Autodesk Inventor part; units mm, degrees
ref_plane "YZ Plane" through (0, 0, 0) normal (1, 0, 0) x (0, 1, 0)
ref_plane "XZ Plane" through (0, 0, 0) normal (0, 1, 0) x (-1, 0, 0)
ref_plane "XY Plane" through (0, 0, 0) normal (0, 0, 1) x (1, 0, 0)
sketch "Эскиз1" plane through (0, 0, 0) normal (0, 0, 1) x (1, 0, 0)
  line L0 (0, 0) -> (10, 0)
  line L1 (10, 0) -> (10, 30)
  line L2 (10, 30) -> (0, 30)
  line L3 (0, 30) -> (0, 0)
  dimension "d0" = 10
  dimension "d1" = 30
revolve "Вращение1" add sketch "Эскиз1" angle 360 about axis through (0, 0, 0) along (1, 0, 0)
sketch "Эскиз2" plane through (0, 0, 0) normal (0, 0, 1) x (1, 0, 0)
  line L0 (0, 0) -> (10, 0)
  line L1 (10, -30) -> (10, 30)
  arc A0 (3, 20) -> (0, 23) centre (0, 20) ccw
  line L2 (3, 20) -> (0, 20) construction
  line L3 (0, 23) -> (0, 20) construction
  line L4 (7, 20) -> (7, 10)
  arc A1 (7, 6) -> (10, 3) centre (10, 6) ccw
  line L5 (7, 6) -> (10, 6) construction
  line L6 (10, 3) -> (10, 6) construction
  arc A2 (10, 23) -> (7, 20) centre (10, 20) ccw
  line L7 (7, 20) -> (10, 20) construction
  line L8 (10, 23) -> (10, 20) construction
  line L9 (7, 10) -> (7, 6)
  line L10 (0, -30) -> (0, 30)
  line L11 (0, 0) -> (0, 23)
  line L12 (10, 3) -> (10, 23)
  line L13 (3, 20) -> (3, 0)
  point P0 (10, 3)
  point P1 (10, 23)
  dimension "d4" = 3
  dimension "d5" = 90
  dimension "d6" = 3
  dimension "d7" = 90
  dimension "d8" = 3
  dimension "d9" = 90
  dimension "d10" = 3
  dimension "d12" = 20
  dimension "d14" = 20
revolve "Вращение2" cut sketch "Эскиз2" angle 360 about axis through (0, 0, 0) along (-1, 0, 0) contours A1 L9 L4 A2 L1
sketch "Эскиз3" plane through (10, 0, 0) normal (1, 0, 0) x (0, 0, -1)
  point P0 (0, 0)
  point P1 (26.5, 0)
  point P2 (13.25, 22.9497)
  point P3 (-13.25, 22.9497)
  point P4 (-26.5, 0)
  point P5 (-13.25, -22.9497)
  point P6 (13.25, -22.9497)
  dimension "d15" = 26.5
  dimension "d18" = 360
hole "Отверстие1" at (10, 0, -26.5) at (10, 22.9497, -13.25) at (10, 22.9497, 13.25) at (10, 0, 26.5) at (10, -22.9497, 13.25) at (10, -22.9497, -13.25) direction (-1, 0, 0) diameter 4 end through all
sketch "Эскиз4" plane through (0, 0, 0) normal (0, 0, 1) x (1, 0, 0)
  line L0 (0, 0) -> (10, 0)
  line L1 (10, 2) -> (10, -2)
  line L2 (0, 0) -> (3, 0)
  line L3 (3, 0) -> (3, 20)
  line L4 (0, 23) -> (0, 23)
  line L5 (0, 23) -> (0, 0)
  arc A0 (10, 23) -> (7, 20) centre (10, 20) ccw construction
  arc A1 (3, 20) -> (0, 23) centre (0, 20) ccw
  dimension "d29" = 3
revolve "Вращение3" cut sketch "Эскиз4" angle 360 about axis through (0, 0, 0) along (1, 0, 0)
equation "\"d25\" = d15"
properties part number "711126 (Доделать)"
Design review of the part built by this model. Coordinates are the model's own, in mm. A direction names the side the tool comes from. Round coordinates to 2 decimals unless told otherwise and drop trailing zeros. Write each loop counter-clockwise with the first axis right and the second up, starting at its lowest first coordinate (ties: lowest second). Pieces come first, ordered by that corner, then holes. Notation, with made-up numbers: M 45.25,79.5 L 53.25,79.5 A24 cw 53.25,95.5 Z; hole C -22.5,77 d8. An arc over 180 degrees is marked long. One line per item, written item: value. Start each with the question number.
1. Take a section at A-A on z = 25.5. State the section outline as (x, y) points, then the cut area to 3 significant figures.
2. For faces 1 (the face through (4.93, -21.733, 14.837)), 2 (the face through (3, 0, 0)), list the 3-axis set-ups (+Z, -Z, +X, -X, +Y, -Y) from which the entire face can be reached by the end or side of a thin tool; tool diameter is ignored.
3. Clearance check with flat-ended pins moving along their axes: P1, Ø3, axis at x = 5, y = -1, coming from the +Z side; P2, Ø1, axis at x = 6, z = -6, coming from the -Y side; P3, Ø4, axis at y = -2, z = 11.5, coming from the -X side. State where each tip first meets the part, or that it passes through.
4. Take a section at C-C on x = 1.25. State the section outline as (y, z) points, then the cut area to 3 significant figures.
5. Take a section at D-D on z = 13.25. State how many separate pieces and enclosed holes the cut face has, then the cut area to 3 significant figures.
6. Take a section at B-B on x = 5.25. State the section outline as (y, z) points, then the cut area to 3 significant figures.
7. Draft analysis for pull direction Z (two halves, no side actions). For faces 3 (the face through (10, 0, 0)), 4 (the face through (7, 4, -5)), 5 (the face through (4.93, -29.97, -1.32)), state which applies: pulls with the +Z half, pulls with the -Z half, needs draft (parallel to the pull), parting line crosses it, or undercut.
8. To check wall thickness, follow probe 1 along Z at (x, y) = (5.5, 0); probe 2 along Z at (x, y) = (1.25, 23); probe 3 along Y at (x, z) = (8.25, 12). State the ranges of each line that lie inside material, in increasing order. Write a range as from..to.
Computed:
1. outline: M 0,-15.8 L 10,-15.8 L 10,-1.73 L 0,-1.73 Z; M 0,1.73 L 10,1.73 L 10,15.8 L 0,15.8 Z
1. area: 281 mm²
2. face 1: +X, -X
2. face 2: -X
3. P1: stops at z = 30
3. P2: stops at y = -29.49
3. P3: stops at x = 3
4. outline: C 0,0 d60; hole C -22.95,-13.25 d4; hole C -22.95,13.25 d4; hole C 0,0 d45.45; hole C 0,-26.5 d4; hole C 0,26.5 d4; hole C 22.95,-13.25 d4; hole C 22.95,13.25 d4
4. area: 1,130 mm²
5. separate pieces: 3
5. enclosed holes: 0
5. area: 242 mm²
6. outline: C 0,0 d60; hole C -22.95,-13.25 d4; hole C -22.95,13.25 d4; hole C 0,-26.5 d4; hole C 0,26.5 d4; hole C 22.95,-13.25 d4; hole C 22.95,13.25 d4
6. area: 2,750 mm²
7. face 3: needs draft
7. face 4: undercut
7. face 5: parting line crosses it
8. probe 1: z = -30..-28.5, -24.5..24.5, 28.5..30
8. probe 2: z = -19.26..-15.25, -11.25..11.25, 15.25..19.26
8. probe 3: y = -27.5..-24.51, -21.39..-18.96, 18.96..21.39, 24.51..27.5
